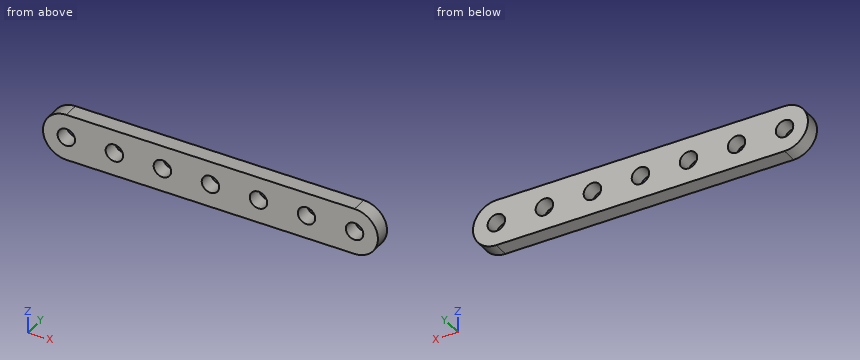
from build123d import *

# Parameters (mm, degrees)
SKETCH1_R           = 1.778
BOSS_EXTRUDE1_DEPTH = 6.35
SKETCH2_W           = 91.819515258
SKETCH2_H           = 20.708231101
CUT_EXTRUDE1_DEPTH  = 3.175


with BuildPart() as part:
    # Sketch1 → Boss-Extrude1 (new body)
    with BuildSketch(Plane.XZ):
        with BuildLine():
            Line((-29.337, -4.7625), (29.337, -4.7625))
            ThreePointArc((29.337, -4.7625), (34.0995, 0), (29.337, 4.7625))
            Line((29.337, 4.7625), (-29.337, 4.7625))
            ThreePointArc((-29.337, 4.7625), (-34.0995, 0), (-29.337, -4.7625))
        make_face()
        with Locations(Location((29.337, 0, 0), (0, 0, 90))):
            Circle(SKETCH1_R, mode=Mode.SUBTRACT)
        with Locations(Location((19.558, 0, 0), (0, 0, 90))):
            Circle(SKETCH1_R, mode=Mode.SUBTRACT)
        with Locations(Location((9.779, 0, 0), (0, 0, 90))):
            Circle(SKETCH1_R, mode=Mode.SUBTRACT)
        with Locations(Location((0, 0, 0), (0, 0, 90))):
            Circle(SKETCH1_R, mode=Mode.SUBTRACT)
        with Locations(Location((-9.779, 0, 0), (0, 0, 90))):
            Circle(SKETCH1_R, mode=Mode.SUBTRACT)
        with Locations(Location((-19.558, 0, 0), (0, 0, 90))):
            Circle(SKETCH1_R, mode=Mode.SUBTRACT)
        with Locations(Location((-29.337, 0, 0), (0, 0, 90))):
            Circle(SKETCH1_R, mode=Mode.SUBTRACT)
    extrude(amount=-BOSS_EXTRUDE1_DEPTH)

    # Sketch2 → Cut-Extrude1 (cut)
    with BuildSketch(Plane(origin=(0, 6.35, 0), x_dir=(1, 0, 0), z_dir=(0, 1, 0))):
        with Locations((-4.688656098, 0.586082012)):
            Rectangle(SKETCH2_W, SKETCH2_H)
    extrude(amount=-CUT_EXTRUDE1_DEPTH, mode=Mode.SUBTRACT)


solid = part.part
Part model, mm, in its own coordinate system. Round coordinates to 2 decimals unless told otherwise and drop trailing zeros. Write each loop counter-clockwise with the first axis right and the second up, starting at its lowest first coordinate (ties: lowest second). Pieces come first, ordered by that corner, then holes. Notation, with made-up numbers: M 60,53 L 94,53 A12 ccw 94,70 Z; hole C 26.25,46 d5. An arc over 180 degrees is marked long. Return JSON: item names as keys, results as strings. Group by question number.
(1) Saw through at C-C on y = 1. Write the cut outline in (x, z) (1 decimal).
(2) Pin check, flat tip, straight feed: pin 1 Ø4.5 at (x, z) = (19.558, 0) entering from -Y. Stop position of the tip, or through.
(3) Saw through at B-B on x = 0. Write the cut outline in (y, z) (1 decimal), then the cut area to 3 significant figures.
(4) Saw through at A-A on z = 0. Count the separate pieces of the cut face and the enclosed holes in it, then the cut area to 4 significant figures.
(5) Saw through at D-D on z = -4. Write the cut outline in (x, y) (3 decimals), then the cut area to 3 significant figures.
(6) Drill centre lines: probe 1 along Z at (x, y) = (9, 2.95); probe 2 along Z at (x, y) = (20.5, 1.8); probe 3 along X at (y, z) = (0.3, 2.5). Where is each one in solid material? Low to high.
Returned:
{
 "1": {"outline": "M -29.3,-4.8 L 29.3,-4.8 A4.8 ccw 29.3,4.8 L -29.3,4.8 A4.8 ccw Z; hole C -29.3,0 d3.6; hole C -19.6,0 d3.6; hole C -9.8,0 d3.6; hole C 0,0 d3.6; hole C 9.8,0 d3.6; hole C 19.6,0 d3.6; hole C 29.3,0 d3.6"},
 "2": {"pin 1": "y = 0"},
 "3": {"outline": "M 0,-4.8 L 3.2,-4.8 L 3.2,-1.8 L 0,-1.8 Z; M 0,1.8 L 3.2,1.8 L 3.2,4.8 L 0,4.8 Z", "area": "19.0 mm²"},
 "4": {"separate pieces": "8", "enclosed holes": "0", "area": "137.5 mm²"},
 "5": {"outline": "M -31.922,0 L 31.922,0 L 31.922,3.175 L -31.922,3.175 Z", "area": "203 mm²"},
 "6": {"probe 1": "-4.76 to -1.6, 1.6 to 4.76", "probe 2": "-4.76 to -1.51, 1.51 to 4.76", "probe 3": "-33.39 to 33.39"}
}
